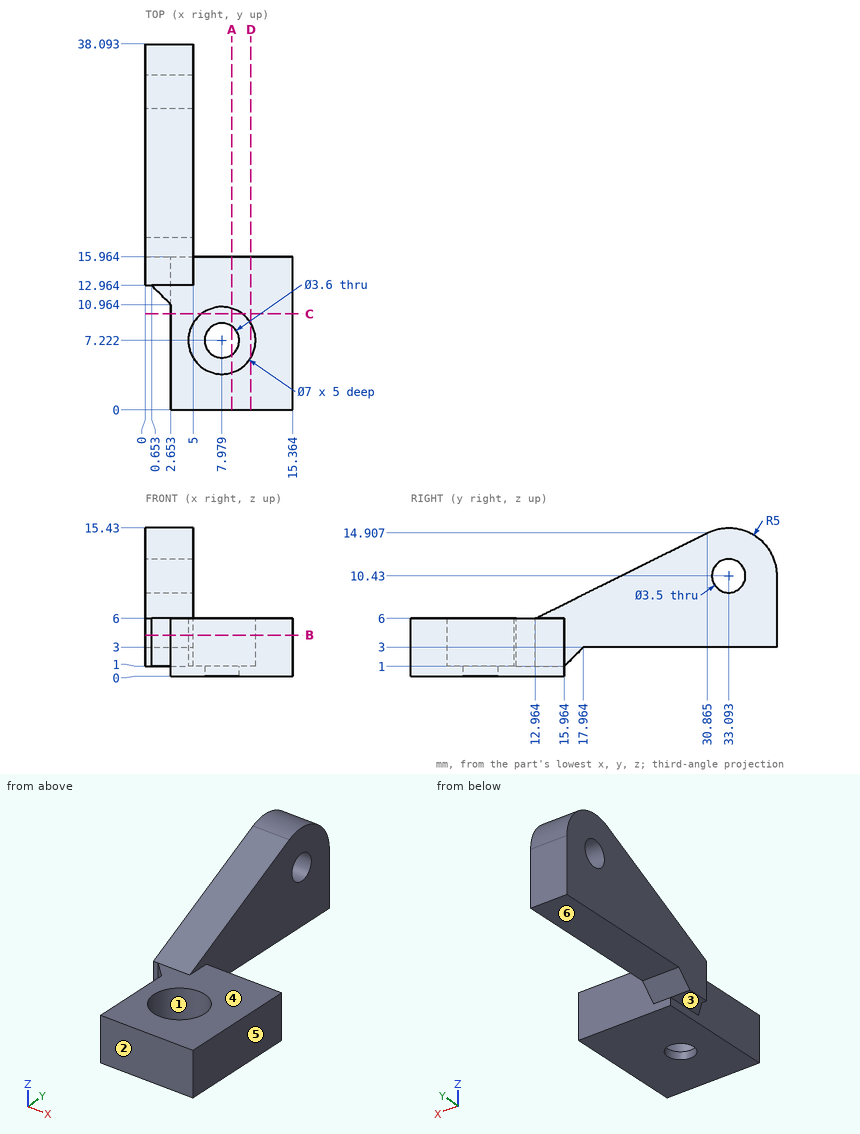
Check sheet for the drawn part. Datum: minimum x, y, z corner. Units: mm. A direction names the side the tool comes from. Coordinates: 2 decimals unless noted, no trailing zeros. Loops run counter-clockwise (first coordinate to the right, second up) from the corner with the lowest first, then second, coordinate; pieces in that order, holes last. Notation, with made-up numbers: M 35,32 L 46,32 A5 cw 46,40 Z; hole C 4.5,7 d3. An arc over 180 degrees is marked long. Answer as a JSON object with one key per item and string values.
1. Sectioned sample at A-A on x = 9. Record the cut outline in (y, z).
Outcome:
{"outline": "M 0,0 L 5.74,0 L 5.74,1 L 3.87,1 L 3.87,6 L 0,6 Z; M 8.7,0 L 15.96,0 L 15.96,6 L 10.57,6 L 10.57,1 L 8.7,1 Z"}
2. Sectioned sample at D-D on x = 11. Record the cut outline in (y, z) (1 decimal).
Outcome:
{"outline": "M 0,0 L 16,0 L 16,6 L 9,6 L 9,1 L 5.5,1 L 5.5,6 L 0,6 Z"}
3. Scan lines: L1, parallel to X at y = 25, z = 11.75; L2, parallel to Y at x = 4.25, z = 11.75 (1 decimal); L3, parallel to Y at x = 2, z = 9.25 (1 decimal). Record each from-to range of solid material in increasing order. Write a range as from..to.
Outcome:
{"L1": "0..5", "L2": "24.5..31.9, 34.2..37.9", "L3": "19.5..31.8, 34.4..38.1"}
4. Sectioned sample at C-C on y = 10. Record the cut outline in (x, z).
Outcome:
{"outline": "M 2.65,0 L 15.36,0 L 15.36,6 L 10.11,6 L 10.11,1 L 5.85,1 L 5.85,6 L 2.65,6 Z"}
5. Access from +Z, -Z, +X, -X, +Y, -Y to the whole of each face (thin tool, end or side, straight path). Record for the marked faces 4, 5 and 6.
Outcome:
{"face 4": "+Z, +X, -Y", "face 5": "+Z, -Z, +X, +Y, -Y", "face 6": "-Z, +X, -X, +Y"}
6. Release check for a two-part mould opening along Y. For the marked faces 1, 2 and 3 record: pulls with the +Y half, pulls with the -Y half, needs draft (parallel to the pull), parting line crosses it, or undercut.
Outcome:
{"face 1": "undercut", "face 2": "pulls with the -Y half", "face 3": "needs draft"}
7. Depth check by flat-ended pin: P1, Ø0.8, axis at x = 1, y = 12.5, coming from the -Z side; P2, Ø2, axis at x = 9, y = 5.5, coming from the +Z side; P3, Ø1.8, axis at y = 11, z = 2.5, coming from the -X side (1 decimal). Enter the tip coordinate at first touch or a pass-through.
Outcome:
{"P1": "z = 1", "P2": "z = 1", "P3": "x = 1.7"}
8. Sectioned sample at B-B on z = 4.25. Record the cut outline in (x, y).
Outcome:
{"outline": "M 0,12.96 L 0.65,12.96 L 2.65,10.96 L 2.65,0 L 15.36,0 L 15.36,15.96 L 5,15.96 L 5,38.09 L 0,38.09 Z; hole C 7.98,7.22 d7"}
